from build123d import *

# Parameters (mm, degrees)
BOSS_EXTRUDE1_DEPTH     = 762
CUT_EXTRUDE1_DEPTH      = 805.176482163
CUT_EXTRUDE2_DEPTH      = 803.239873394
CUT_EXTRUDE2_DEPTH_BACK = 803.239873394
SKETCH4_R               = 2.5
CUT_EXTRUDE3_DEPTH      = 773.997626217
CUT_EXTRUDE3_DEPTH_BACK = 773.997626217
SKETCH5_R               = 7.5
SKETCH5_R_2             = 2.5


with BuildPart() as part:
    # Sketch2 → Boss-Extrude1 (new body)
    with BuildSketch(Plane.XY):
        with BuildLine():
            Line((-28.176229758, 236.761091532), (-124.876229758, 236.761091532))
            ThreePointArc((-124.876229758, 236.761091532), (-126.997550102, 235.882411875), (-127.876229758, 233.761091532))
            Line((-127.876229758, 233.761091532), (-127.876229758, 216.761091532))
            ThreePointArc((-127.876229758, 216.761091532), (-126.997550102, 214.639771188), (-124.876229758, 213.761091532))
            Line((-124.876229758, 213.761091532), (-102.417718129, 213.761091532))
            Line((-102.417718129, 213.761091532), (-93.418737463, 219.298462014))
            Line((-93.418737463, 219.298462014), (-83.376229758, 213.761091532))
            Line((-83.376229758, 213.761091532), (-47.876229758, 213.761091532))
            ThreePointArc((-47.876229758, 213.761091532), (-45.754909415, 214.639771188), (-44.876229758, 216.761091532))
            Line((-44.876229758, 216.761091532), (-44.876229758, 232.461091532))
            ThreePointArc((-44.876229758, 232.461091532), (-44.788361793, 232.673223566), (-44.576229758, 232.761091532))
            Line((-44.576229758, 232.761091532), (-28.176229758, 232.761091532))
            ThreePointArc((-28.176229758, 232.761091532), (-27.964097724, 232.848959498), (-27.876229758, 233.061091532))
            Line((-27.876229758, 233.061091532), (-27.876229758, 236.461091532))
            ThreePointArc((-27.876229758, 236.461091532), (-27.964097724, 236.673223566), (-28.176229758, 236.761091532))
        make_face()
        with BuildLine():
            Line((-49.176229758, 234.761091532), (-92.576229758, 234.761091532))
            ThreePointArc((-92.576229758, 234.761091532), (-92.788361793, 234.673223566), (-92.876229758, 234.461091532))
            Line((-92.876229758, 234.461091532), (-92.876229758, 221.283213521))
            Line((-92.876229758, 221.283213521), (-82.861376535, 215.761091532))
            Line((-82.861376535, 215.761091532), (-50.876229758, 215.761091532))
            ThreePointArc((-50.876229758, 215.761091532), (-49.462016196, 216.34687797), (-48.876229758, 217.761091532))
            Line((-48.876229758, 217.761091532), (-48.876229758, 234.461091532))
            ThreePointArc((-48.876229758, 234.461091532), (-48.964097724, 234.673223566), (-49.176229758, 234.761091532))
        make_face(mode=Mode.SUBTRACT)
        with BuildLine():
            Line((-95.176229758, 234.761091532), (-122.376229758, 234.761091532))
            ThreePointArc((-122.376229758, 234.761091532), (-123.43688993, 234.321751704), (-123.876229758, 233.261091532))
            Line((-123.876229758, 233.261091532), (-123.876229758, 217.261091532))
            ThreePointArc((-123.876229758, 217.261091532), (-123.43688993, 216.20043136), (-122.376229758, 215.761091532))
            Line((-122.376229758, 215.761091532), (-104.891920236, 215.761091532))
            Line((-104.891920236, 215.761091532), (-94.876229758, 221.924077192))
            Line((-94.876229758, 221.924077192), (-94.876229758, 234.461091532))
            ThreePointArc((-94.876229758, 234.461091532), (-94.964097724, 234.673223566), (-95.176229758, 234.761091532))
        make_face(mode=Mode.SUBTRACT)
    extrude(amount=BOSS_EXTRUDE1_DEPTH)

    # Sketch3 → Cut-Extrude1 (cut, through all)
    with BuildSketch(Plane.ZY.offset(127.876229758)):
        Polygon((0, 236.761091532), (23, 213.761091532), (0, 213.761091532), align=None)
        Polygon((762, 236.761091532), (739, 213.761091532), (762, 213.761091532), align=None)
    extrude(amount=-CUT_EXTRUDE1_DEPTH, mode=Mode.SUBTRACT)

    # Sketch4 → Cut-Extrude2 (cut, two sides: drawn at the far end of the back side and taken through both)
    with BuildSketch(Plane(origin=(-44.876229758, 0, 0), x_dir=(0, 0, -1), z_dir=(1, 0, 0)).offset(-CUT_EXTRUDE2_DEPTH_BACK)):
        with Locations(Location((-700.4, 225.961091532, 0), (0, 0, 180))):
            Circle(SKETCH4_R)
        with Locations(Location((-675, 225.961091532, 0), (0, 0, 180))):
            Circle(SKETCH4_R)
        with Locations(Location((-649.6, 225.961091532, 0), (0, 0, 180))):
            Circle(SKETCH4_R)
        with Locations(Location((-624.2, 225.961091532, 0), (0, 0, 180))):
            Circle(SKETCH4_R)
        with Locations(Location((-137.8, 225.961091532, 0), (0, 0, 180))):
            Circle(SKETCH4_R)
        with Locations(Location((-112.4, 225.961091532, 0), (0, 0, 180))):
            Circle(SKETCH4_R)
        with Locations(Location((-87, 225.961091532, 0), (0, 0, 180))):
            Circle(SKETCH4_R)
        with Locations(Location((-61.6, 225.961091532, 0), (0, 0, 180))):
            Circle(SKETCH4_R)
    extrude(amount=CUT_EXTRUDE2_DEPTH + CUT_EXTRUDE2_DEPTH_BACK, mode=Mode.SUBTRACT)

    # Sketch5 → Cut-Extrude3 (cut, two sides: drawn at the far end of the back side and taken through both)
    with BuildSketch(Plane(origin=(0, 236.761091532, 0), x_dir=(1, 0, 0), z_dir=(0, 1, 0)).offset(-CUT_EXTRUDE3_DEPTH_BACK)):
        with Locations(Location((-78.026229758, -381, 0), (0, 0, 229.857845338))):
            Circle(SKETCH5_R)
        with Locations(Location((-78.026229758, -351, 0), (0, 0, 270))):
            Circle(SKETCH5_R_2)
        with Locations(Location((-78.026229758, -411, 0), (0, 0, 270))):
            Circle(SKETCH5_R_2)
    extrude(amount=CUT_EXTRUDE3_DEPTH + CUT_EXTRUDE3_DEPTH_BACK, mode=Mode.SUBTRACT)


solid = part.part
For this review, take the finished solid that the model builds, in its own axes (mm). A direction names the side the tool comes from. Round coordinates to 2 decimals unless told otherwise and drop trailing zeros. Loops run counter-clockwise (first coordinate to the right, second up) from the corner with the lowest first, then second, coordinate; pieces in that order, holes last. Notation, with made-up numbers: (34, -24) - (39, -24) arc R21 cw to (39, -10) - close; hole circle Ø8 at (-31.75, 1). An arc over 180 degrees is marked (long way). Use one line per item in the form item = value.
1) We need section A-A on x = -113.5. Write out the cut boundary in (y, z).
Solutions:
outline = (213.76, 23) - (215.76, 21) - (215.76, 741) - (213.76, 739) - close; (234.76, 2) - (236.76, 0) - (236.76, 762) - (234.76, 760) - close
2) Mouldability with a two-part tool opening along Z and no side actions: class faces 1 (the face through (-85.52, 235.54, 760.78)), 2 (the face through (-80.92, 215.17, 387.92)), 3 (the face through (-70.588, 235.747, 380.042)), 4 (the face through (-127.876, 225, 376)) as pulls with the +Z half, pulls with the -Z half, needs draft (parallel to the pull), parting line crosses it, or undercut.
Solutions:
face_1 = pulls with the +Z half
face_2 = undercut
face_3 = undercut
face_4 = needs draft
3) Clearance check with flat-ended pins moving along their axes: P1, Ø6, axis at y = 230, z = 149.5, coming from the +X side; P2, Ø6.5, axis at y = 225.96, z = 675, coming from the +X side; P3, Ø4.5, axis at y = 225.96, z = 112.4, coming from the -X side; P4, Ø3, axis at x = -99.5, z = 112, coming from the -Y side. State where each tip first meets the part, or that it passes through.
Solutions:
P1 = -27.88
P2 = -44.88
P3 = through
P4 = 214.63
4) Tool access review of faces 5 (the face through (-44.876, 225, 376)), 6 (the face through (-66, 213.761, 376)), 7 (the face through (-48.876, 226, 376)): name each direction out of +Z, -Z, +X, -X, +Y, -Y from which nothing blocks a thin tool from reaching the whole face with its end or side.
Solutions:
face_5 = +Z, -Z, +X, -Y
face_6 = +Z, -Z, +X, -X, -Y
face_7 = +Z, -Z
5) We need section B-B on z = 195.5. State how many separate pieces and enclosed holes the cut face has, then the cut area to 3 significant figures.
Solutions:
separate_pieces = 1
enclosed_holes = 2
area = 592 mm2
6) Wall thickness on probe 1 along X at (y, z) = (229.25, 301); probe 2 along X at (y, z) = (233.75, 151); probe 3 along Y at (x, z) = (-67, 452): over which ranges is each line inside the solid? List them lowest first.
Solutions:
probe_1 = -127.88 to -123.88, -94.88 to -92.88, -48.88 to -44.88
probe_2 = -127.88 to -123.79, -94.88 to -92.88, -48.88 to -27.88
probe_3 = 213.76 to 215.76, 234.76 to 236.76
